Can you work these out from the drawing? Everything is in mm from the part's minimum corner. A direction names the side the tool comes from. Round coordinates to 2 decimals unless told otherwise and drop trailing zeros. Loops run counter-clockwise (first coordinate to the right, second up) from the corner with the lowest first, then second, coordinate; pieces in that order, holes last. Notation, with made-up numbers: M 38.25,78.5 L 62.25,78.5 A11 cw 62.25,82.5 Z; hole C -34,23 d7. An arc over 180 degrees is marked long. Answer in a Markdown table with one row per item.
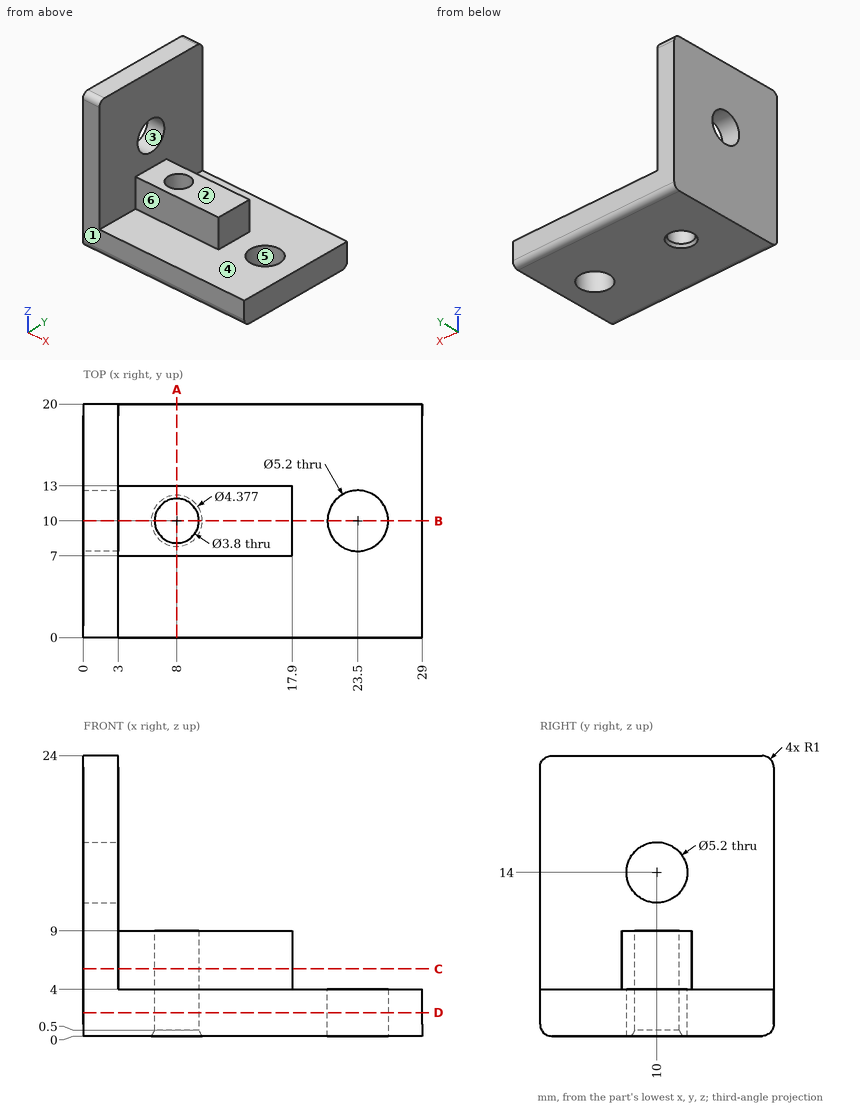
1) I want a section at D-D, the plane z = 2. Please give me the cut outline in (x, y).
Computed:
| item | result |
|---|---|
| outline | M 0,0 L 29,0 L 29,20 L 0,20 Z; hole C 8,10 d3.8; hole C 23.5,10 d5.2 |
2) Will these pins go through, and if not, where does the flat tip stop? P1, Ø4, axis at y = 10, z = 14, coming from the -X side; P2, Ø5, axis at x = 23.5, y = 12.5, coming from the +Z side; P3, Ø1.5, axis at x = 9.5, z = 7, coming from the -Y side; P4, Ø6, axis at x = 19, y = 11, coming from the +Z side.
Computed:
| item | result |
|---|---|
| P1 | passes through |
| P2 | stops at z = 4 |
| P3 | stops at y = 7 |
| P4 | stops at z = 9 |
3) I want a section at B-B, the plane y = 10. Please give me the cut outline in (x, z), plus the area to 3 significant figures.
Computed:
| item | result |
|---|---|
| outline | M 0,0 L 5.81,0 L 6.1,0.5 L 6.1,9 L 3,9 L 3,11.4 L 0,11.4 Z; M 0,16.6 L 3,16.6 L 3,24 L 0,24 Z; M 9.9,0.5 L 10.19,0 L 20.9,0 L 20.9,4 L 17.9,4 L 17.9,9 L 9.9,9 Z; M 26.1,0 L 29,0 L 29,4 L 26.1,4 Z |
| area | 180 mm² |
4) I need wall thicknesses on line 1 (Z direction, x = 2.35, y = 10); line 2 (Z direction, x = 20.25, y = 18.75); line 3 (Z direction, x = 6.25, y = 11.5). Which ranges of each line are inside material? Lowest first, please.
Computed:
| item | result |
|---|---|
| line 1 | z = 0 to 11.4, 16.6 to 24 |
| line 2 | z = 0 to 4 |
| line 3 | z = 0 to 9 |
5) Which directions (+Z, -Z, +X, -X, +Y, -Y) give clear straight access to the entire face, cutting with the end or side of a thin tool? Please do the marked faces 1 and 2.
Computed:
| item | result |
|---|---|
| face 1 | +Z, -Z, +X, -X, -Y |
| face 2 | +Z, +X, +Y, -Y |
6) If we mould it in two halves opening along Y, with no side actions, what happens to the marked faces 3, 4, 5 and 6? For each: released by +Y, released by -Y, zero draft, split by the parting line, or undercut.
Computed:
| item | result |
|---|---|
| face 3 | undercut |
| face 4 | zero draft |
| face 5 | undercut |
| face 6 | released by -Y |
7) I want a section at A-A, the plane x = 8. Please give me the cut outline in (y, z).
Computed:
| item | result |
|---|---|
| outline | M 0,1 A1 ccw 1,0 L 7.81,0 L 8.1,0.5 L 8.1,9 L 7,9 L 7,4 L 0,4 Z; M 11.9,0.5 L 12.19,0 L 19,0 A1 ccw 20,1 L 20,4 L 13,4 L 13,9 L 11.9,9 Z |
8) I want a section at C-C, the plane z = 5.75. Please give me the cut outline in (x, y), plus the area to 3 significant figures.
Computed:
| item | result |
|---|---|
| outline | M 0,0 L 3,0 L 3,7 L 17.9,7 L 17.9,13 L 3,13 L 3,20 L 0,20 Z; hole C 8,10 d3.8 |
| area | 138 mm² |
